from build123d import *

# Parameters (mm, degrees)
BOSS_EXTRUDE1_DEPTH = 5
CUT_EXTRUDE1_DEPTH  = 10
SKETCH4_W           = 17
SKETCH4_H           = 10
BOSS_EXTRUDE3_DEPTH = 5
FILLET1_R           = 3


with BuildPart() as part:
    # Sketch1 → Boss-Extrude1 (new body)
    with BuildSketch(Plane.XY):
        Polygon((0, 0), (127.279220614, 0), (127.279220614, 10), (106.066017178, 31.213203436), (102.530483272, 27.67766953), (81.317279836, 48.890872965), (84.852813742, 52.426406871), (63.639610307, 73.639610307), (42.426406871, 52.426406871), (45.961940777, 48.890872965), (24.748737342, 27.67766953), (21.213203436, 31.213203436), (0, 10), align=None)
    extrude(amount=BOSS_EXTRUDE1_DEPTH)

    # Sketch2 → Cut-Extrude1 (cut)
    with BuildSketch(Plane.XY.offset(5)):
        Polygon((127.279220614, 3), (121.279220614, 3), (121.279220614, 1.5), (117.279220614, 1.5), (117.279220614, 3), (115.279220614, 3), (115.279220614, 7), (117.279220614, 7), (117.279220614, 8.5), (121.279220614, 8.5), (121.279220614, 7), (127.279220614, 7), align=None)
        Polygon((36.769552622, 39.69848481), (33.941125497, 36.870057685), (38.183766184, 32.627416998), (37.123106012, 31.566756826), (39.951533137, 28.738329701), (41.012193309, 29.798989873), (42.426406871, 28.384776311), (45.254833996, 31.213203436), (43.840620434, 32.627416998), (44.901280605, 33.68807717), (42.072853481, 36.516504294), (41.012193309, 35.455844123), align=None)
        Polygon((0, 7), (0, 3), (6, 3), (6, 1.5), (10, 1.5), (10, 3), (12, 3), (12, 7), (10, 7), (10, 8.5), (6, 8.5), (6, 7), align=None)
        Polygon((48.639610307, 5), (61.639610307, 5), (61.639610307, 11), (60.139610307, 11), (60.139610307, 15), (61.639610307, 15), (61.639610307, 17), (65.639610307, 17), (65.639610307, 15), (67.139610307, 15), (67.139610307, 11), (65.639610307, 11), (65.639610307, 5), (78.639610307, 5), (78.639610307, 0), (48.639610307, 0), align=None)
        Polygon((93.338095117, 36.870057685), (89.09545443, 32.627416998), (90.156114601, 31.566756826), (87.327687477, 28.738329701), (86.267027305, 29.798989873), (84.852813742, 28.384776311), (82.024386618, 31.213203436), (83.43860018, 32.627416998), (82.377940008, 33.68807717), (85.206367133, 36.516504294), (86.267027305, 35.455844123), (90.509667992, 39.69848481), align=None)
    extrude(amount=-CUT_EXTRUDE1_DEPTH, mode=Mode.SUBTRACT)

    # Sketch4 → Boss-Extrude3 (add)
    with BuildSketch(Plane.XY.offset(5)):
        with Locations((8.5, -5)):
            Rectangle(SKETCH4_W, SKETCH4_H)
        with Locations((118.779220614, -5)):
            Rectangle(SKETCH4_W, SKETCH4_H)
    extrude(amount=-BOSS_EXTRUDE3_DEPTH)

    # Fillet1
    fillet1_edges = [part.edges().sort_by_distance(p)[0] for p in [
        (17, 0, 2.5),
        (17, -10, 2.5),
        (110.279220614, -10, 2.5),
        (110.279220614, 0, 2.5),
    ]]
    fillet(fillet1_edges, radius=FILLET1_R)


solid = part.part
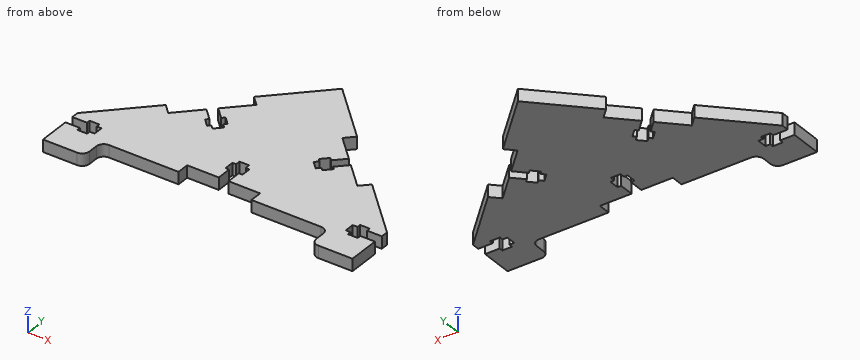
Part model, mm, in its own coordinate system. Coordinates: 2 decimals unless noted, no trailing zeros. Order: outer loops, then holes, each group sorted by start corner. A loop starts at its lowest first (then second) coordinate and runs counter-clockwise, first axis right, second up.
(1) Probe L1, parallel to Y at x = 43.5, z = 3.15; L2, parallel to X at y = 9, z = 0.2; L3, parallel to X at y = -4.5, z = 4.7. List the from-to ranges inside material, lowest first.
Check sheet entries:
L1: y = 0 to 29.46, 35.09 to 46.43, 51.35 to 53.5
L2: x = 0 to 61.64, 65.64 to 127.28
L3: x = 0 to 17, 110.28 to 127.28
(2) Slice it at C-C, the plane x = 71.5. Write the cut outline in (y, z).
Check sheet entries:
outline: (5, 0) - (65.78, 0) - (65.78, 5) - (5, 5) - close
(3) Slice it at A-A, the plane x = 8.5. Write the cut outline in (y, z), and give its area (4 significant figures).
Check sheet entries:
outline: (-10, 0) - (1.5, 0) - (1.5, 5) - (-10, 5) - close; (8.5, 0) - (18.5, 0) - (18.5, 5) - (8.5, 5) - close
area: 107.5 mm2
(4) Pin check, flat tips, straight feed: pin 1 Ø1 at (x, z) = (98.5, 2.5) entering from +Y; pin 2 Ø3 at (y, z) = (14, 3.5) entering from +X; pin 3 Ø3 at (x, z) = (73, 2.5) entering from +Y. Stop position of each tip, or through.
Check sheet entries:
pin 1: stops at y = 32.21
pin 2: stops at x = 124.78
pin 3: stops at y = 65.78
(5) Slice it at B-B, the plane y = 60. Write the cut outline in (x, z), and give its area (3 significant figures).
Check sheet entries:
outline: (50, 0) - (77.28, 0) - (77.28, 5) - (50, 5) - close
area: 136 mm2
